```python
from build123d import *

# Parameters (mm, degrees)
SKETCH1_W           = 37.5
SKETCH1_H           = 93
SKETCH1_W_2         = 33.5
SKETCH1_H_2         = 89
BOSS_EXTRUDE1_DEPTH = 5
SKETCH2_W           = 40
SKETCH2_H           = 100
SKETCH2_W_2         = 33.5
SKETCH2_H_2         = 89
BOSS_EXTRUDE2_DEPTH = 4
SKETCH3_W           = 37.5
SKETCH3_H           = 93
SKETCH3_W_2         = 33.5
SKETCH3_H_2         = 89
BOSS_EXTRUDE3_DEPTH = 5
SKETCH4_R           = 6
CUT_EXTRUDE1_DEPTH  = 5
SKETCH5_R           = 3.5
CUT_EXTRUDE2_DEPTH  = 5


with BuildPart() as part:
    # Sketch1 → Boss-Extrude1 (new body)
    with BuildSketch(Plane(origin=(0, 0, 0), x_dir=(1, 0, 0), z_dir=(0, 1, 0))):
        Rectangle(SKETCH1_W, SKETCH1_H)
        Rectangle(SKETCH1_W_2, SKETCH1_H_2, mode=Mode.SUBTRACT)
    extrude(amount=BOSS_EXTRUDE1_DEPTH)

    # Sketch2 → Boss-Extrude2 (add)
    with BuildSketch(Plane(origin=(0, 5, 0), x_dir=(1, 0, 0), z_dir=(0, 1, 0))):
        Rectangle(SKETCH2_W, SKETCH2_H)
        Rectangle(SKETCH2_W_2, SKETCH2_H_2, mode=Mode.SUBTRACT)
    extrude(amount=BOSS_EXTRUDE2_DEPTH)

    # Sketch3 → Boss-Extrude3 (add)
    with BuildSketch(Plane(origin=(0, 9, 0), x_dir=(1, 0, 0), z_dir=(0, 1, 0))):
        Rectangle(SKETCH3_W, SKETCH3_H)
        Rectangle(SKETCH3_W_2, SKETCH3_H_2, mode=Mode.SUBTRACT)
    extrude(amount=BOSS_EXTRUDE3_DEPTH)

    # Sketch4 → Cut-Extrude1 (cut)
    with BuildSketch(Plane(origin=(0, 0, -46.5), x_dir=(-1, 0, 0), z_dir=(0, 0, -1))):
        with Locations((-11.5, -3)):
            Circle(SKETCH4_R)
    extrude(amount=-CUT_EXTRUDE1_DEPTH, mode=Mode.SUBTRACT)

    # Sketch5 → Cut-Extrude2 (cut)
    with BuildSketch(Plane(origin=(0, 0, -46.5), x_dir=(-1, 0, 0), z_dir=(0, 0, -1))):
        with Locations((10.5, -1)):
            Circle(SKETCH5_R)
    extrude(amount=-CUT_EXTRUDE2_DEPTH, mode=Mode.SUBTRACT)


solid = part.part
```
Geometry: final body of the model. Coordinates: model frame, mm. A direction names the side the tool comes from. Coordinates: 2 decimals unless noted, no trailing zeros. Order: outer loops, then holes, each group sorted by start corner. A loop starts at its lowest first (then second) coordinate and runs counter-clockwise, first axis right, second up.
Item 1: Section query D-D (y = 6). Output: boundary loops of the cut face in (x, z).
Answer:
outline: (-20, -50) - (20, -50) - (20, 50) - (-20, 50) - close; hole (-16.75, -44.5) - (16.75, -44.5) - (16.75, 44.5) - (-16.75, 44.5) - close
Item 2: Material intervals for line 1 along X through (y, z) = (4.25, 10.5); line 2 along Z through (x, y) = (1, 8); line 3 along X through (y, z) = (8.25, -14.5), sorted ascending.
Answer:
line 1: x = -18.75 to -16.75, 16.75 to 18.75
line 2: z = -50 to -44.5, 44.5 to 50
line 3: x = -20 to -16.75, 16.75 to 20
Item 3: Draft query along Z for faces 1 (the face through (0, 11, -46.5)), 2 (the face through (0, 7, -44.5)), 3 (the face through (-18.75, 11, 1)). Return one class per face: released by +Z, released by -Z, zero draft, split by the parting line, or undercut.
Answer:
face 1: released by -Z
face 2: undercut
face 3: zero draft
Item 4: Contact query for flat-ended pins moving along their axis: P1, Ø2.5, axis at y = 3, z = 22.5, coming from the +X side; P2, Ø5, axis at y = 12.5, z = -26, coming from the -X side; P3, Ø2.5, axis at x = -7.5, y = 12.5, coming from the -Z side; P4, Ø5.5, axis at y = 11, z = -20, coming from the -X side. Output: stop coordinate, or through.
Answer:
P1: stops at x = 18.75
P2: stops at x = -18.75
P3: stops at z = -46.5
P4: stops at x = -20
Item 5: Section query B-B (z = -19). Output: boundary loops of the cut face in (x, y).
Answer:
outline: (-20, 5) - (-18.75, 5) - (-18.75, 0) - (-16.75, 0) - (-16.75, 14) - (-18.75, 14) - (-18.75, 9) - (-20, 9) - close; (16.75, 0) - (18.75, 0) - (18.75, 5) - (20, 5) - (20, 9) - (18.75, 9) - (18.75, 14) - (16.75, 14) - close
Item 6: Section query C-C (y = 10.75). Output: boundary loops of the cut face in (x, z).
Answer:
outline: (-18.75, -46.5) - (18.75, -46.5) - (18.75, 46.5) - (-18.75, 46.5) - close; hole (-16.75, -44.5) - (16.75, -44.5) - (16.75, 44.5) - (-16.75, 44.5) - close
Item 7: Section query A-A (x = -3). Output: boundary loops of the cut face in (y, z).
Answer:
outline: (0, -46.5) - (5, -46.5) - (5, -50) - (9, -50) - (9, -46.5) - (14, -46.5) - (14, -44.5) - (0, -44.5) - close; (0, 44.5) - (14, 44.5) - (14, 46.5) - (9, 46.5) - (9, 50) - (5, 50) - (5, 46.5) - (0, 46.5) - close
Item 8: Access query for faces 4 (the face through (0, 3, -46.5)), 5 (the face through (0, 2, 46.5)), 6 (the face through (0, 11, 46.5)), 7 (the face through (0, 7, 44.5)), 8 (the face through (-10.6, 2.5, -45.5)). Directions: +Z, -Z, +X, -X, +Y, -Y. A direction counts if a zero-diameter tool reaches every point of the face in a straight line with its end or side. Return the directions, or none.
Answer:
face 4: -Z, +X, -X, -Y
face 5: +Z, +X, -X, -Y
face 6: +Z, +X, -X, +Y
face 7: +Y, -Y
face 8: -Z, -Y
